CAD build for the part. Positions are in the model's coordinates, mm. Face numbers are marked on the shaded views. A direction names the side the tool comes from. Round coordinates to 2 decimals unless told otherwise and drop trailing zeros. Write each loop counter-clockwise with the first axis right and the second up, starting at its lowest first coordinate (ties: lowest second). Pieces come first, ordered by that corner, then holes. Notation, with made-up numbers: (-35.75, 26.5) - (-10.75, 26.5) arc R17 ccw to (-10.75, 58.5) - close; hole circle Ø3 at (-2, -6). An arc over 180 degrees is marked (long way). Use one line per item in the form item = value. Start each with the question number.
Item 1: Band-saw the part on D-D, the plane x = 3. List the corners of the cut face in (y, z), and give its area (3 significant figures).
Item 2: Band-saw the part on B-B, the plane x = 12. List the corners of the cut face in (y, z).
Item 3: Pin check, flat tips, straight feed: pin 1 (6 mm diameter, centred on x = 11.5, z = 16, fed in from +Y); pin 2 (10 mm diameter, centred on x = 9, z = 46.5, fed in from +Y); pin 3 (2 mm diameter, centred on x = 0.5, y = 1, fed in from -Z). Stop position of each tip, or through.
Item 4: Pull direction Z, two halves, no side cores. Call the marked faces 4, 5 and 6: +Z half, -Z half, draft (parallel to the pull), parting line (faces both ways), or undercut.
Item 5: Band-saw the part on A-A, the plane z = 48. List the corners of the cut face in (x, y), and give its area (4 significant figures).
Item 6: Drill centre lines: L1, parallel to X at y = -20.5, z = 48.5; L2, parallel to Y at x = 24.5, z = 59; L3, parallel to Z at x = -4, y = -5. Where is each one in solid material? Low to high.
Item 7: Tool access for the marked faces 1, 2 and 3: list every direction of +Z, -Z, +X, -X, +Y, -Y with a clear straight run to the whole face (end or side of a thin tool).
Item 8: Band-saw the part on C-C, the plane y = 13. List the corners of the cut face in (x, z).
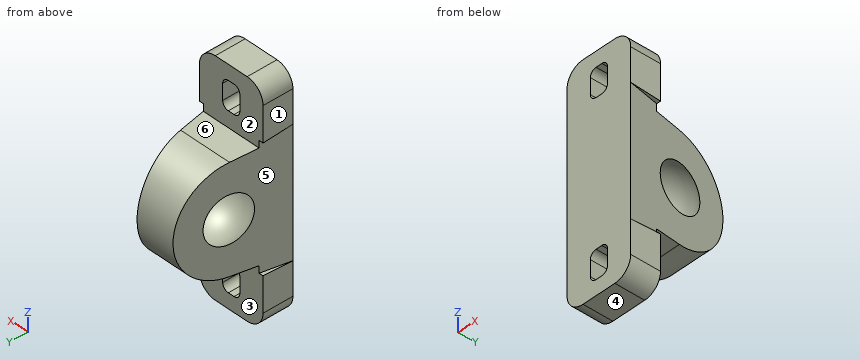
Solid Edge part; units mm, degrees
sketch "Sketch1" plane through (0, -30.2, 0) normal (0, -1, 0) x (1, 0, 0)
  line L0 (-8, -54.75) -> (-8, 54.75)
  arc A0 (-8, 54.75) -> (1.75, 64.5) centre (1.75, 54.75) cw
  line L1 (1.75, 64.5) -> (21.25, 64.5)
  arc A1 (21.25, 64.5) -> (31, 54.75) centre (21.25, 54.75) cw
  line L2 (31, 54.75) -> (31, -54.75)
  arc A2 (31, -54.75) -> (21.25, -64.5) centre (21.25, -54.75) cw
  line L3 (21.25, -64.5) -> (1.75, -64.5)
  arc A3 (1.75, -64.5) -> (-8, -54.75) centre (1.75, -54.75) cw
  line L4 (6.25, 43.5) -> (6.25, 52.5)
  arc A4 (6.25, 52.5) -> (9.75, 56) centre (9.75, 52.5) cw
  line L5 (9.75, 56) -> (13.25, 56)
  arc A5 (13.25, 56) -> (16.75, 52.5) centre (13.25, 52.5) cw
  line L6 (16.75, 52.5) -> (16.75, 43.5)
  arc A6 (16.75, 43.5) -> (13.25, 40) centre (13.25, 43.5) cw
  line L7 (13.25, 40) -> (9.75, 40)
  arc A7 (9.75, 40) -> (6.25, 43.5) centre (9.75, 43.5) cw
  arc A8 (6.25, -43.5) -> (9.75, -40) centre (9.75, -43.5) cw
  line L8 (9.75, -40) -> (13.25, -40)
  arc A9 (13.25, -40) -> (16.75, -43.5) centre (13.25, -43.5) cw
  line L9 (16.75, -43.5) -> (16.75, -52.5)
  arc A10 (16.75, -52.5) -> (13.25, -56) centre (13.25, -52.5) cw
  line L10 (13.25, -56) -> (9.75, -56)
  arc A11 (9.75, -56) -> (6.25, -52.5) centre (9.75, -52.5) cw
  line L11 (6.25, -52.5) -> (6.25, -43.5)
extrude "ExtrudedProtrusion_1" add sketch "Sketch1" against normal blind 17
sketch "Sketch2" plane through (11.5, 0, 0) normal (1, 0, 0) x (0, 1, 0)
  line L0 (-30.2, 32) -> (-30.2, -32)
  line L1 (-30.2, -32) -> (1.7464, -30.1495)
  arc A0 (1.7464, -30.1495) -> (1.7464, 30.1495) centre (0, 0) ccw
  line L2 (1.7464, 30.1495) -> (-30.2, 32)
extrude "ExtrudedProtrusion_2" add sketch "Sketch2" against normal blind 19.5 and the other way blind 19.5
sketch "Sketch3" plane through (31, 0, 0) normal (1, 0, 0) x (0, 1, 0)
  line L0 (-30.2, 36) -> (1.9707, 34.1432)
  arc A0 (1.9707, 34.1432) -> (1.9707, -34.1432) centre (0, 0) cw
  line L1 (1.9707, -34.1432) -> (-30.2, -36)
  line L2 (-30.2, -36) -> (-30.2, 36)
revolve "RevolvedCutout_1" cut sketch "Sketch3" angle 8 about axis through (31, -30.2, -36) along (0, 0, 1)
sketch "Sketch4" plane through (-8, 0, 0) normal (1, 0, 0) x (0, 1, 0)
  line L0 (-30.2, 36) -> (1.9707, 34.1432)
  arc A0 (1.9707, 34.1432) -> (1.9707, -34.1432) centre (0, 0) cw
  line L1 (1.9707, -34.1432) -> (-30.2, -36)
  line L2 (-30.2, -36) -> (-30.2, 36)
revolve "RevolvedCutout_2" cut sketch "Sketch4" angle 8 about axis through (-8, -30.2, -36) along (0, 0, -1)
sketch "Sketch5" plane through (0, 0, 0) normal (0, 0, 1) x (1, 0, 0)
  arc A0 (31.5, 0) -> (-8.5, 0) centre (11.5, 0) cw
  line L0 (-8.5, 0) -> (31.5, 0)
revolve "RevolvedCutout1" cut sketch "Sketch5" angle 360 about axis through (-8.5, 0, 0) along (1, 0, 0)
properties part number "UCP201 GB/T7810-1995_PART5"
Determined:
q1.outline = (-30.2, -64.5) - (-13.2, -64.5) - (-13.2, -31.02) - (1.75, -30.15) arc R30.2 ccw to (1.75, 30.15) - (-13.2, 31.02) - (-13.2, 64.5) - (-30.2, 64.5) - close; hole circle Ø36.21 at (0, 0)
q1.area = 3,400 mm²
q2.outline = (-30.2, -64.5) - (-13.2, -64.5) - (-13.2, -56) - (-30.2, -56) - close; (-30.2, -40) - (-13.2, -40) - (-13.2, -31.02) - (1.75, -30.15) arc R30.2 ccw to (1.75, 30.15) - (-13.2, 31.02) - (-13.2, 40) - (-30.2, 40) - close; (-30.2, 56) - (-13.2, 56) - (-13.2, 64.5) - (-30.2, 64.5) - close; hole circle Ø39.99 at (0, 0)
q3.pin_1 = 27.26
q3.pin_2 = -13.2
q3.pin_3 = -30.25
q4.face_4 = -Z half
q4.face_5 = undercut
q4.face_6 = +Z half
q5.outline = (-8, -30.2) - (6.25, -30.2) - (6.25, -13.2) - (-8, -13.2) - close; (16.75, -30.2) - (31, -30.2) - (31, -13.2) - (16.75, -13.2) - close
q5.area = 484.5 mm²
q6.L1 = -8 to 6.25, 16.75 to 31
q6.L2 = -30.2 to -13.2
q6.L3 = -30.54 to -11.61, 11.61 to 30.54
q7.face_1 = +Z, -Z, -X, +Y, -Y
q7.face_2 = +Z, +X, -X, +Y
q7.face_3 = -Z, +X, -X, +Y
q8.outline = (-1.93, -27.26) - (24.93, -27.26) - (24.93, -7.12) arc R15.2 cw to (-1.93, -7.12) - close; (-1.93, 7.12) arc R15.2 cw to (24.93, 7.12) - (24.93, 27.26) - (-1.93, 27.26) - close
